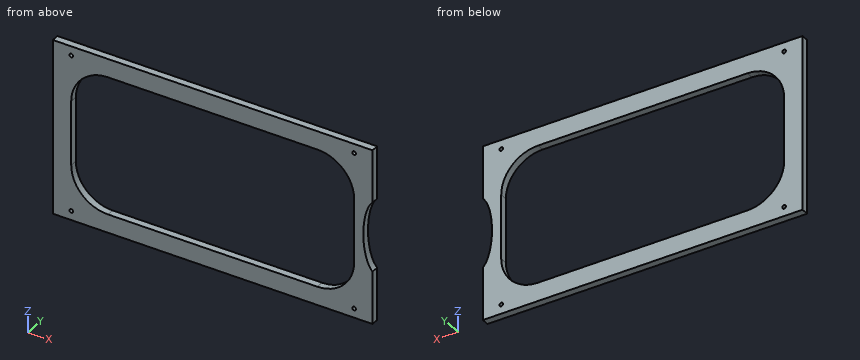
from build123d import *

# Parameters (mm, degrees)
F0_W     = 220.98
F0_H     = 120.65
F1_DEPTH = 5.08
F3_DEPTH = 5.081
F4_R     = 1.27
F5_DEPTH = 5.081


with BuildPart() as f1:
    # F0 (on Front) → F1 (new body)
    with BuildSketch(Plane.XZ):
        with Locations((110.49, 60.325)):
            Rectangle(F0_W, F0_H)
    extrude(amount=F1_DEPTH)

    # F2 (on face) → F3 (cut, through all)
    with BuildSketch(Plane.XZ.offset(5.08)):
        with BuildLine():
            Line((12.7, 82.55), (12.7, 38.1))
            ThreePointArc((12.7, 38.1), (20.139488, 20.139488), (38.1, 12.7))
            Line((38.1, 12.7), (182.88, 12.7))
            ThreePointArc((182.88, 12.7), (200.840512, 20.139488), (208.28, 38.1))
            Line((208.28, 38.1), (208.28, 82.55))
            ThreePointArc((208.28, 82.55), (200.840512, 100.510512), (182.88, 107.95))
            Line((182.88, 107.95), (38.1, 107.95))
            ThreePointArc((38.1, 107.95), (20.139488, 100.510512), (12.7, 82.55))
        make_face()
    extrude(amount=-F3_DEPTH, mode=Mode.SUBTRACT)

    # F4 (on face) → F5 (cut, through all)
    with BuildSketch(Plane.XZ.offset(5.08)):
        with Locations((12.7, 114.3)):
            Circle(F4_R)
        with Locations((12.7, 6.35)):
            Circle(F4_R)
        with Locations((208.28, 114.3)):
            Circle(F4_R)
        with Locations((208.28, 6.35)):
            Circle(F4_R)
        with BuildLine():
            add(Edge.make_bspline(
                [(224.155, 85.725), (207.657216, 85.725), (215.906108, 47.625), (224.155, 9.525), (232.403892, 47.625), (240.652784, 85.725), (224.155, 85.725)],
                knots=[0, 0, 0, 2.094395, 2.094395, 4.18879, 4.18879, 6.283185, 6.283185, 6.283185], degree=2, weights=[1, 0.5, 1, 0.5, 1, 0.5, 1]))
        make_face()
    extrude(amount=-F5_DEPTH, mode=Mode.SUBTRACT)


solid = f1.part
CAD build for the part. Positions are in the model's coordinates, mm. Coordinates: 2 decimals unless noted, no trailing zeros. Write each loop counter-clockwise with the first axis right and the second up, starting at its lowest first coordinate (ties: lowest second). Pieces come first, ordered by that corner, then holes. Notation, with made-up numbers: (65.25, 6) - (84.25, 6) arc R21 ccw to (84.25, 28) - close; hole circle Ø2 at (9, 14.25). An arc over 180 degrees is marked (long way). Use a Markdown table: item, result. Add a question column.
Item 1: Band-saw the part on A-A, the plane x = 108. Give the cut face in (y, z), and give its area (3 significant figures).
Item 2: Flat gauge pins, fed straight in: pin 1 (2.5 mm diameter, centred on x = 123.5, y = -3.5, fed in from -Z); pin 2 (2.5 mm diameter, centred on y = -3, z = 68.5, fed in from +X). Where does each tip first touch, or does it go through?
Item 3: Band-saw the part on B-B, the plane z = 105. Give the cut face in (x, y).
Item 4: Band-saw the part on C-C, the plane y = -2.4. Give the number of separate pieces and of enclosed holes in the cut face, and give its area (3 significant figures).
Item 5: Drill centre lines: L1, parallel to X at y = -4.25, z = 6; L2, parallel to X at y = -3.3, z = 114.3; L3, parallel to Z at x = 137, y = -4.4. Where is each one in solid material? Low to high. Write a range as from..to.
Numbers:
| question | item | result |
|---|---|---|
| 1 | outline | (-5.08, 0) - (0, 0) - (0, 12.7) - (-5.08, 12.7) - close; (-5.08, 107.95) - (0, 107.95) - (0, 120.65) - (-5.08, 120.65) - close |
| 1 | area | 129 mm2 |
| 2 | pin 1 | z = 0 |
| 2 | pin 2 | x = 215.31 |
| 3 | outline | (0, -5.08) - (26.22, -5.08) - (26.22, 0) - (0, 0) - close; (194.76, -5.08) - (220.98, -5.08) - (220.98, 0) - (194.76, 0) - close |
| 4 | separate pieces | 1 |
| 4 | enclosed holes | 5 |
| 4 | area | 8,340 mm2 |
| 5 | L1 | 0..11.48, 13.92..207.06, 209.5..220.98 |
| 5 | L2 | 0..11.43, 13.97..207.01, 209.55..220.98 |
| 5 | L3 | 0..12.7, 107.95..120.65 |
